Source: CAD feature listing. Evaluate the final solid. Frame: model axes, mm. Face numbers are marked on the shaded views. A direction names the side the tool comes from. Round coordinates to 2 decimals unless told otherwise and drop trailing zeros. Order: outer loops, then holes, each group sorted by start corner. A loop starts at its lowest first (then second) coordinate and runs counter-clockwise, first axis right, second up.
```python
from build123d import *

# Parameters (mm, degrees)
SKETCH1_R           = 3.5
BOSS_EXTRUDE1_DEPTH = 33
SKETCH2_R           = 2.6
BOSS_EXTRUDE2_DEPTH = 3.19
BOSS_EXTRUDE3_DEPTH = 7.5
SKETCH5_W           = 3.4
SKETCH5_H           = 3.4
BOSS_EXTRUDE4_DEPTH = 7.5


with BuildPart() as part:
    # Sketch1 → Boss-Extrude1 (new body)
    with BuildSketch(Plane(origin=(0, 0, 0), x_dir=(1, 0, 0), z_dir=(0, 1, 0))):
        with Locations(Location((0, 0, 0), (0, 0, 270))):
            Circle(SKETCH1_R)
    extrude(amount=BOSS_EXTRUDE1_DEPTH)

    # Sketch2 → Boss-Extrude2 (add)
    with BuildSketch(Plane(origin=(0, 33, 0), x_dir=(1, 0, 0), z_dir=(0, 1, 0))):
        with Locations(Location((0, 0, 0), (0, 0, 90))):
            Circle(SKETCH2_R)
    extrude(amount=BOSS_EXTRUDE2_DEPTH)

    # Sketch4 → Boss-Extrude3 (add)
    with BuildSketch(Plane(origin=(0, 36.19, 0), x_dir=(1, 0, 0), z_dir=(0, 1, 0))):
        with BuildLine():
            Line((1.758185656, -1.915406798), (1.758185656, 1.915406798))
            ThreePointArc((1.758185656, 1.915406798), (-0.216604889, 2.59096166), (-2.051814344, 1.59689007))
            Line((-2.051814344, 1.59689007), (-2.051814344, -1.59689007))
            ThreePointArc((-2.051814344, -1.59689007), (-0.216604889, -2.59096166), (1.758185656, -1.915406798))
        make_face()
    extrude(amount=BOSS_EXTRUDE3_DEPTH)

    # Loft2: read off the stored shape, not the designer's step
    # Loft2: loft between two sections, ruled curve by curve
    loft2_from = [
        Edge.make_bspline([(0.603918101, 33, 3.447503869), (7.498925839, 33, 2.239667668), (6.291089638, 33, -4.65534007), (-0.603918101, 33, -3.447503869), (-7.498925839, 33, -2.239667668), (-6.291089638, 33, 4.65534007), (0.603918101, 33, 3.447503869)], [0, 0, 0, 0, 0.5, 0.5, 0.5, 1, 1, 1, 1], 3, [1, 0.333333333, 0.333333333, 1, 0.333333333, 0.333333333, 1]),
    ]
    loft2_to = [
        Edge.make_bspline([(1.447224244, 36.19, 2.123780118), (5.694784479, 36.19, -0.77066837), (2.800335991, 36.19, -5.018228605), (-1.447224244, 36.19, -2.123780118), (-5.694784479, 36.19, 0.77066837), (-2.800335991, 36.19, 5.018228605), (1.447224244, 36.19, 2.123780118)], [0, 0, 0, 0, 0.5, 0.5, 0.5, 1, 1, 1, 1], 3, [1, 0.333333333, 0.333333333, 1, 0.333333333, 0.333333333, 1]),
    ]
    loft2 = Solid(Shell([*[Face.make_surface_from_curves(loft2_from[k], loft2_to[k]) for k in range(1)], Face(Wire(loft2_from)), Face(Wire(loft2_to))]))
    add(loft2)

    # Sketch5 → Boss-Extrude4 (add)
    with BuildSketch(Plane.XZ):
        Rectangle(SKETCH5_W, SKETCH5_H)
    extrude(amount=BOSS_EXTRUDE4_DEPTH)


solid = part.part
```
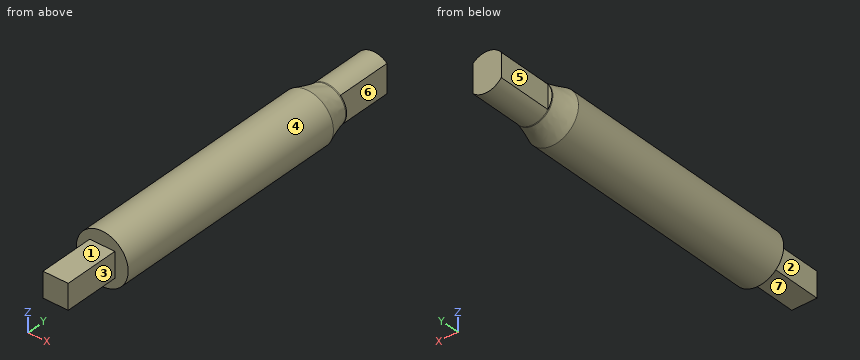
1. Pull-direction query (X, two-part tool) for the marked faces 1, 2, 3 and 4; classes: released by +X, released by -X, zero draft, split by the parting line, or undercut.
2. Line query: line 1 along X through (y, z) = (-4, -1.25); line 2 along Y through (x, z) = (0.75, -1.75); line 3 along Z through (x, y) = (-0.25, 24). Output: solid intervals per line, ascending.
3. Section B-B on y = 7. Return loops of the section in (x, z), plus the area to 3 significant figures.
4. First-contact query: pin 1 (1.5 mm diameter, centred on y = 19, z = -2, fed in from +X); pin 2 (3.5 mm diameter, centred on y = 39, z = 0, fed in from -X); pin 3 (1.7 mm diameter, centred on y = -2.5, z = -0.5, fed in from -X). Flat tips, straight axial feed; report the tip coordinate or a pass-through.
5. Section A-A on y = -0.5. Return loops of the section in (x, z).
6. Access query for the marked faces 5, 6 and 7. Directions: +Z, -Z, +X, -X, +Y, -Y. A direction counts if a zero-diameter tool reaches every point of the face in a straight line with its end or side. Return the directions, or none.
Result:
1. face 1: zero draft
1. face 2: released by -X
1. face 3: released by +X
1. face 4: split by the parting line
2. line 1: x = -1.7 to 1.7
2. line 2: y = 0 to 43.69
2. line 3: z = -3.49 to 3.49
3. outline: circle Ø7 at (0, 0)
3. area: 38.5 mm2
4. pin 1: stops at x = 3.27
4. pin 2: stops at x = -2.05
4. pin 3: stops at x = -1.7
5. outline: (-1.7, -1.7) - (1.7, -1.7) - (1.7, 1.7) - (-1.7, 1.7) - close
6. face 5: +Z, -Z, -X, +Y
6. face 6: +Z, -Z, +X, +Y
6. face 7: -Z, +X, -X, -Y
